```python
from build123d import *

# Parameters (mm, degrees)
SKETCH1_W                = 18
SKETCH1_H                = 110
BOSS_EXTRUDE1_DEPTH      = 46
BOSS_EXTRUDE2_DEPTH      = 27
FILLET1_R                = 30
BOSS_EXTRUDE3_DEPTH      = 6
BOSS_EXTRUDE3_DEPTH_BACK = 60
SKETCH3_R                = 30
FILLET3_R                = 20
SKETCH4_W                = 18
SKETCH4_H                = 50
CUT_EXTRUDE1_DEPTH       = 170.764542823
HOLE1_D                  = 36
HOLE2_D                  = 16
RIB1_REACH               = 195.184
SKETCH9_WALL_W           = 446.367700514
SKETCH9_WALL_H           = 12


with BuildPart() as part:
    # Sketch1 → Boss-Extrude1 (new, symmetric)
    with BuildSketch(Plane(origin=(0, 0, 0), x_dir=(0, 0, -1), z_dir=(1, 0, 0))):
        with Locations((9, 55)):
            Rectangle(SKETCH1_W, SKETCH1_H)
    extrude(amount=BOSS_EXTRUDE1_DEPTH, both=True)

    # Sketch2 → Boss-Extrude2 (add, symmetric)
    with BuildSketch(Plane(origin=(0, 0, 0), x_dir=(0, 0, -1), z_dir=(1, 0, 0))):
        Polygon((0, 0), (-18, 0), (-18, 48), (-78, 48), (-78, 0), (-152, 0), (-152, 60), (-40, 60), (-40, 68), (0, 68), align=None)
    extrude(amount=BOSS_EXTRUDE2_DEPTH, both=True)

    # Fillet1
    fillet1_edges = [part.edges().sort_by_distance(p)[0] for p in [
        (0, 0, 152),
        (0, 60, 152),
    ]]
    fillet(fillet1_edges, radius=FILLET1_R - 0.0001)  # a hair under: the kernel refuses the full size

    # Sketch3 → Boss-Extrude3 (add, two sides: drawn at the far end of the back side and taken through both)
    with BuildSketch(Plane(origin=(27, 0, 0), x_dir=(0, 0, -1), z_dir=(1, 0, 0)).offset(-BOSS_EXTRUDE3_DEPTH_BACK)):
        with Locations((-122, 30)):
            Circle(SKETCH3_R)
    extrude(amount=BOSS_EXTRUDE3_DEPTH + BOSS_EXTRUDE3_DEPTH_BACK)

    # Fillet3
    fillet3_edges = [part.edges().sort_by_distance(p)[0] for p in [
        (46, 110, -9),
        (-46, 110, -9),
    ]]
    fillet(fillet3_edges, radius=FILLET3_R)

    # Sketch4 → Cut-Extrude1 (cut, through all)
    with BuildSketch(Plane(origin=(0, 60, 0), x_dir=(1, 0, 0), z_dir=(0, 1, 0))):
        with Locations((0, -127)):
            Rectangle(SKETCH4_W, SKETCH4_H)
    extrude(amount=-CUT_EXTRUDE1_DEPTH, mode=Mode.SUBTRACT)

    # Hole1 (through all)
    with Locations(Plane(origin=(33, 0, 0), x_dir=(0, 0, -1), z_dir=(1, 0, 0))):
        with Locations((-122, 30)):
            Hole(HOLE1_D / 2)

    # Hole2 (through all)
    with Locations(Plane.XY):
        with Locations((26, 90), (-26, 90)):
            Hole(HOLE2_D / 2)

    # Sketch9 wall → Rib1 (add, up to next)
    with BuildSketch(Plane(origin=(0, 89, 20), x_dir=(0, -0.724137931034, 0.689655172414), z_dir=(0, -0.689655172414, -0.724137931034)), mode=Mode.PRIVATE) as rib1_sk1:
        Rectangle(SKETCH9_WALL_W, SKETCH9_WALL_H)
    rib1_tool1 = extrude(rib1_sk1.sketch, amount=RIB1_REACH, mode=Mode.PRIVATE) - part.part
    add(rib1_tool1.solids().sort_by_distance((0, 89, 20))[0])


solid = part.part
```
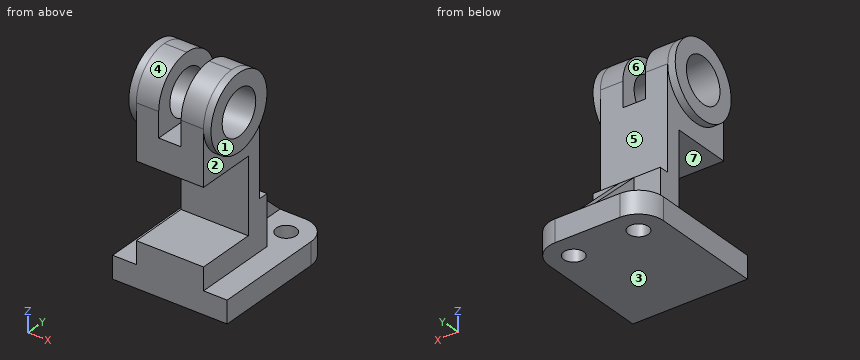
The listing builds one solid part. Answer for the finished solid, in the listing's coordinates (mm). Face numbers are marked on the shaded views. A direction names the side the tool comes from. Give positions to 0.01 mm unless a question says otherwise; leave off trailing zeros. Order: outer loops, then holes, each group sorted by start corner. A loop starts at its lowest first (then second) coordinate and runs counter-clockwise, first axis right, second up. Notation, with made-up numbers: M 58.5,-3 L 71.5,-3 A30 cw 71.5,28 Z; hole C 33,62 d11. An arc over 180 degrees is marked long. Put each result on its own line as item: value. Start each with the question number.
Item 1: The part is cut by section D-D, the plane x = -29.5. Determine the outline of the cut face in (y, z), and give its area (3 significant figures).
Item 2: Find the intervals of material crossed by line 1 along Z through (x, y) = (-32, 39); line 2 along Y through (x, z) = (26.5, 122); line 3 along Z through (x, y) = (10, 103.5), in increasing order.
Item 3: Flat-ended cylindrical pins translate along their axes: P1, Ø3, axis at x = -28.5, z = 131, coming from the +Y side; P2, Ø18.5, axis at x = -26, y = 90, coming from the +Z side; P3, Ø1, axis at x = 0, y = 74.5, coming from the +Z side; P4, Ø21, axis at x = 26, y = 90, coming from the -Z side. Find the tip coordinate at first contact, or state that the pin passes through.
Item 4: The part is cut by section B-B, the plane y = 17. State how many separate pieces and enclosed holes the cut face has, and give its area (3 significant figures).
Item 5: The part is cut by section C-C, the plane x = 0. Determine the outline of the cut face in (y, z), and give its area (3 significant figures).
Item 6: For a pull along Z with two mould halves and no side action, classify the marked faces 1, 2, 3 and 4 as +Z half, -Z half, draft (parallel to the pull), parting line (faces both ways), or undercut.
Item 7: The part is cut by section A-A, the plane z = 2. Determine the outline of the cut face in (x, y).
Item 8: Which of the six approach directions +Z, -Z, +X, -X, +Y, -Y give full straight-line access (tool end or side, diameter ignored) to the marked faces 5, 6 and 7?
Answer key:
1. outline: M 0,-18 L 82.81,-18 L 82.81,0 L 0,0 Z; C 30,122 d60; M 97.19,-18 L 109.69,-18 L 109.69,0 L 97.19,0 Z; hole C 30,122 d36
1. area: 3,530 mm²
2. line 1: z = -18 to 0, 93.38 to 106.41, 137.59 to 150.62
2. line 2: y = 0 to 12, 48 to 60
2. line 3: z = -18 to 0
3. P1: stops at y = 59.05
3. P2: stops at z = 0
3. P3: stops at z = 34.29
3. P4: stops at z = -18
4. separate pieces: 4
4. enclosed holes: 0
4. area: 5,070 mm²
5. outline: M 0,-18 L 110,-18 L 110,0 L 68,40 L 60,40 L 60,102 L 0,102 L 0,78 L 48,78 L 48,18 L 0,18 Z
5. area: 6,380 mm²
6. face 1: draft
6. face 2: undercut
6. face 3: -Z half
6. face 4: +Z half
7. outline: M -27,0 L 27,0 L 27,68 L 6,68 L 6,107.9 L -6,107.9 L -6,68 L -27,68 Z
8. face 5: +Z, +X, -X, +Y
8. face 6: +Z, +Y, -Y
8. face 7: +X, -X, -Y
